The drawing under review shows one solid part. Ordinate dimensions are in mm from its lowest x, y, z. A direction names the side the tool comes from. Coordinates: 2 decimals unless noted, no trailing zeros. Order: outer loops, then holes, each group sorted by start corner. A loop starts at its lowest first (then second) coordinate and runs counter-clockwise, first axis right, second up. Notation, with made-up numbers: (67.5, 10.25) - (85.5, 10.25) arc R22 ccw to (85.5, 17.25) - close; hole circle Ø7 at (-39, 51). An arc over 180 degrees is marked (long way). Answer in a Markdown table with one row per item.
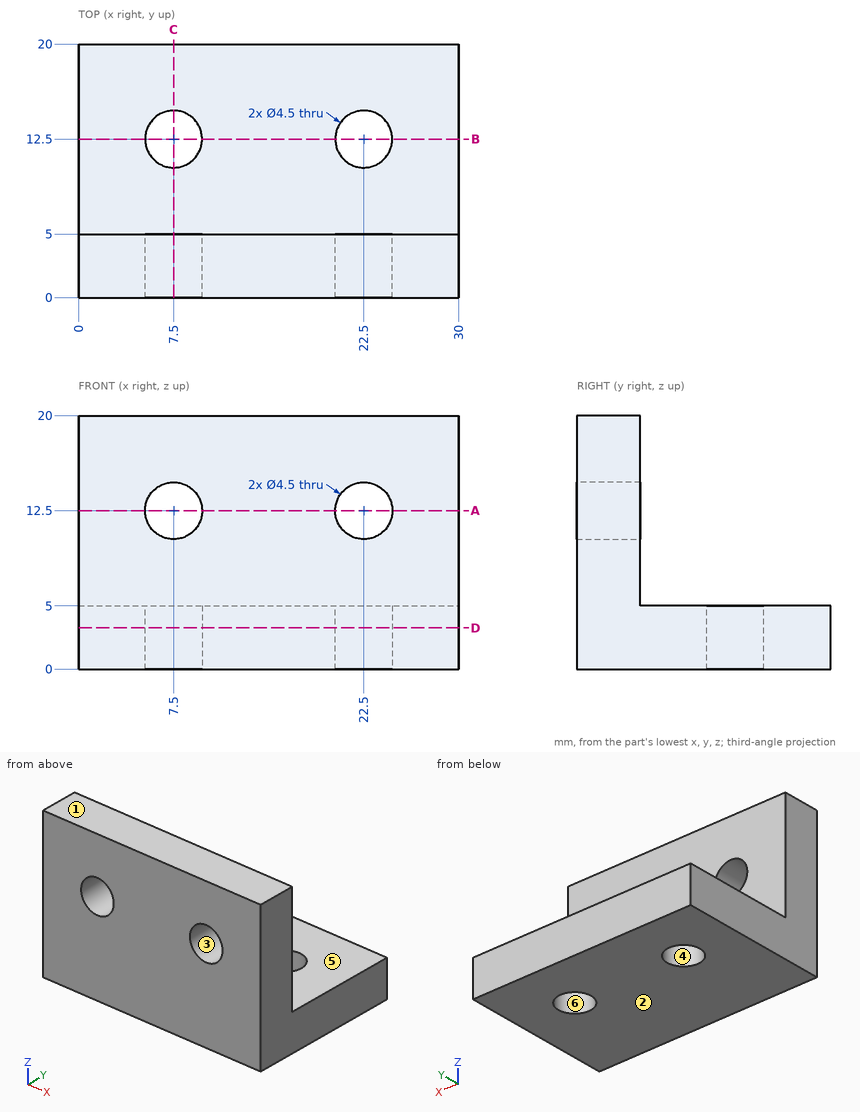
Item 1: We need section D-D, the plane z = 3.25. Write out the cut boundary in (x, y), then the cut area to 3 significant figures.
Check values:
| item | result |
|---|---|
| outline | (0, 0) - (30, 0) - (30, 20) - (0, 20) - close; hole circle Ø4.5 at (7.5, 12.5); hole circle Ø4.5 at (22.5, 12.5) |
| area | 568 mm^2 |
Item 2: We need section C-C, the plane x = 7.5. Write out the cut boundary in (y, z).
Check values:
| item | result |
|---|---|
| outline | (0, 0) - (10.25, 0) - (10.25, 5) - (5, 5) - (5, 10.25) - (0, 10.25) - close; (0, 14.75) - (5, 14.75) - (5, 20) - (0, 20) - close; (14.75, 0) - (20, 0) - (20, 5) - (14.75, 5) - close |
Item 3: We need section A-A, the plane z = 12.5. Write out the cut boundary in (x, y).
Check values:
| item | result |
|---|---|
| outline | (0, 0) - (5.25, 0) - (5.25, 5) - (0, 5) - close; (9.75, 0) - (20.25, 0) - (20.25, 5) - (9.75, 5) - close; (24.75, 0) - (30, 0) - (30, 5) - (24.75, 5) - close |
Item 4: Mouldability with a two-part tool opening along Z and no side actions: class the marked faces 1, 2, 3 and 4 as +Z half, -Z half, draft (parallel to the pull), parting line (faces both ways), or undercut.
Check values:
| item | result |
|---|---|
| face 1 | +Z half |
| face 2 | -Z half |
| face 3 | undercut |
| face 4 | draft |
Item 5: To check wall thickness, follow line 1 (X direction, y = 2, z = 12.5); line 2 (Y direction, x = 7.5, z = 2.8); line 3 (Z direction, x = 13, y = 14). State the ranges of each line that lie inside material, in increasing order. Write a range as from..to.
Check values:
| item | result |
|---|---|
| line 1 | 0..5.25, 9.75..20.25, 24.75..30 |
| line 2 | 0..10.25, 14.75..20 |
| line 3 | 0..5 |
Item 6: Clearance check with flat-ended pins moving along their axes: pin 1 Ø12 at (x, y) = (14, 8.5) entering from -Z; pin 2 Ø2 at (x, z) = (25, 17.5) entering from +Y; pin 3 Ø5 at (x, y) = (7.5, 12.5) entering from +Z. State where each tip first meets the part, or that it passes through.
Check values:
| item | result |
|---|---|
| pin 1 | z = 0 |
| pin 2 | y = 5 |
| pin 3 | z = 5 |
Item 7: Tool access review of the marked faces 5 and 6: name each direction out of +Z, -Z, +X, -X, +Y, -Y from which nothing blocks a thin tool from reaching the whole face with its end or side.
Check values:
| item | result |
|---|---|
| face 5 | +Z, +X, -X, +Y |
| face 6 | +Z, -Z |
